The listing builds one solid part. Answer for the finished solid, in the listing's coordinates (mm). Face numbers are marked on the shaded views. A direction names the side the tool comes from. Coordinates: 2 decimals unless noted, no trailing zeros. Order: outer loops, then holes, each group sorted by start corner. A loop starts at its lowest first (then second) coordinate and runs counter-clockwise, first axis right, second up. Notation, with made-up numbers: (84.25, 76) -> (90.25, 76) arc R15 ccw to (90.25, 87) -> close; hole circle Ø4 at (69, -2.5). An arc over 180 degrees is marked (long way). Put each result on its own line as item: value. Start each with the question number.
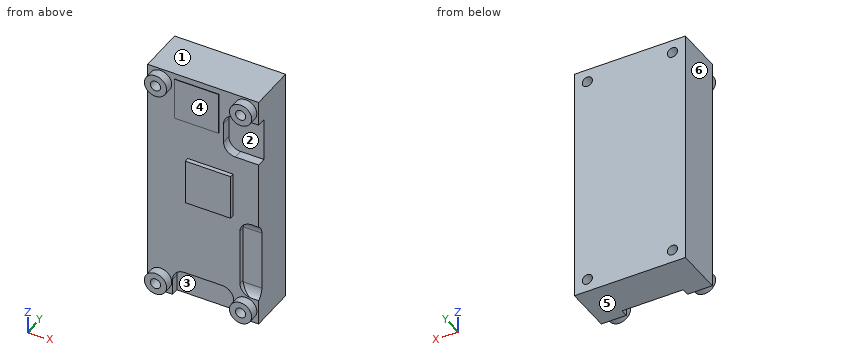
Autodesk Inventor part; units mm, degrees
ref_plane "YZ Plane" through (0, 0, 0) normal (1, 0, 0) x (0, 1, 0)
ref_plane "XZ Plane" through (0, 0, 0) normal (0, 1, 0) x (-1, 0, 0)
ref_plane "XY Plane" through (0, 0, 0) normal (0, 0, 1) x (1, 0, 0)
sketch "Sketch1" plane through (0, 0, 0) normal (0, 1, 0) x (-1, 0, 0)
  line L0 (15, 32.5) -> (-15, 32.5)
  line L1 (-15, 32.5) -> (-15, -32.5)
  line L2 (-15, -32.5) -> (15, -32.5)
  line L3 (15, -32.5) -> (15, 32.5)
  point P0 (0, 0)
  dimension "d0" = 65
  dimension "d1" = 30
  dimension "d2" = 15
  dimension "d3" = 32.5
extrude "Extrusion1" add sketch "Sketch1" along normal blind 12.7
sketch "Sketch2" plane through (0, 0, 0) normal (0, -1, 0) x (1, 0, 0)
  line L0 (8.07, 8.904) -> (-4.13, 8.904)
  line L1 (-4.13, 8.904) -> (-4.13, -3.296)
  line L2 (-4.13, -3.296) -> (8.07, -3.296)
  line L3 (8.07, -3.296) -> (8.07, 8.904)
  line L4 (-15, 32.5) -> (15, 32.5)
  line L5 (15, 32.5) -> (15, -32.5)
  point P0 (0, 0)
  dimension "d6" = 12.2
  dimension "d7" = 12.2
  dimension "d8" = 23.596
  dimension "d9" = 6.93
extrude "Extrusion2" add sketch "Sketch2" along normal blind 1.17
sketch "Sketch3" plane through (0, 0, 0) normal (0, -1, 0) x (1, 0, 0)
  line L0 (15, 32.5) -> (15, -32.5)
  line L1 (15, 25.85) -> (5.5, 25.85)
  line L2 (5.5, 25.85) -> (5.5, 14.15)
  line L3 (5.5, 14.15) -> (15, 14.15)
  line L4 (15, 14.15) -> (15, 25.85)
  line L5 (-15, 32.5) -> (15, 32.5)
  point P0 (0, 0)
  dimension "d12" = 9.5
  dimension "d13" = 11.7
  dimension "d14" = 6.65
extrude "Extrusion3" cut sketch "Sketch3" against normal blind 2.5
sketch "Sketch4" plane through (0, 0, 0) normal (0, -1, 0) x (1, 0, 0)
  line L0 (15, 14.15) -> (15, -32.5)
  line L1 (15, -4.75) -> (10.3, -4.75)
  line L2 (10.3, -4.75) -> (10.3, -13.05)
  line L3 (10.3, -13.05) -> (15, -13.05)
  line L4 (15, -13.05) -> (15, -4.75)
  line L5 (-15, 32.5) -> (15, 32.5)
  point P0 (0, 0)
  dimension "d17" = 4.7
  dimension "d18" = 8.3
  dimension "d19" = 37.25
extrude "Extrusion4" cut sketch "Sketch4" against normal blind 1
sketch "Sketch5" plane through (0, 0, 0) normal (0, -1, 0) x (1, 0, 0)
  line L0 (15, -13.05) -> (15, -32.5)
  line L1 (10.3, -25.65) -> (15, -25.65)
  line L2 (15, -32.5) -> (-15, -32.5)
  line L3 (10.3, -4.75) -> (15, -4.75)
  line L4 (15, -25.65) -> (15, -4.115)
  line L5 (15, -4.115) -> (9.92, -4.115)
  line L6 (9.92, -4.115) -> (9.92, -25.65)
  line L7 (10.3, -25.65) -> (9.92, -25.65)
  point P0 (0, 0)
  point P1 (15, -7.29)
  dimension "d22" = 4.7
  dimension "d24" = 6.85
  dimension "d69" = 5.08
  dimension "d70" = 0.635
extrude "Extrusion5" cut sketch "Sketch5" against normal blind 1.5
sketch "Sketch6" plane through (0, 0, 0) normal (0, -1, 0) x (1, 0, 0)
  circle A0 centre (11.5, 29) radius 3
  circle A1 centre (-11.5, 29) radius 3
  circle A2 centre (-11.5, -29) radius 3
  circle A3 centre (11.5, -29) radius 3
  line L0 (15, -32.5) -> (-15, -32.5)
  line L1 (-15, -32.5) -> (-15, 32.5)
  line L2 (-15, 32.5) -> (15, 32.5)
  point P0 (0, 0)
  dimension "d27" = 6
  dimension "d28" = 6
  dimension "d29" = 6
  dimension "d30" = 6
  dimension "d31" = 0
  dimension "d32" = 23
  dimension "d33" = 58
  dimension "d34" = 3.5
  dimension "d35" = 23
  dimension "d37" = 0
  dimension "d38" = 3.5
  dimension "d42" = 3.5
extrude "Extrusion6" add sketch "Sketch6" along normal blind 2.42
sketch "Sketch7" plane through (11.5, -2.42, 29) normal (0, -1, 0) x (1, 0, 0)
  circle A0 centre (0, 0) radius 3
  circle A1 centre (0, -58) radius 3
  circle A2 centre (-23, -58) radius 3
  circle A3 centre (-23, 0) radius 3
  point P0 (-11.5, -29)
hole "Hole1" at (11.5, -2.42, 29) at (-11.5, -2.42, 29) at (-11.5, -2.42, -29) at (11.5, -2.42, -29) direction (0, 1, 0) diameter 2.75 depth 25.4 tip angle 118
sketch "Sketch8" plane through (0, 0, 0) normal (0, -1, 0) x (1, 0, 0)
  line L0 (15, -32.5) -> (-15, -32.5)
  line L1 (8.255, -32.5) -> (-8.255, -32.5)
  line L2 (-8.255, -32.5) -> (-8.255, -24.88)
  line L3 (-8.255, -24.88) -> (8.255, -24.88)
  line L4 (8.255, -24.88) -> (8.255, -32.5)
  point P0 (0, 0)
  point P1 (0, 0)
  dimension "d50" = 7.62
  dimension "d51" = 16.51
  dimension "d52" = 8.255
extrude "Extrusion7" cut sketch "Sketch8" against normal blind 2.032
sketch "Sketch9" plane through (0, 0, 0) normal (0, -1, 0) x (1, 0, 0)
  line L0 (4.228, 30.9) -> (-7.722, 30.9)
  line L1 (-7.722, 30.9) -> (-7.722, 19.5)
  line L2 (-7.722, 19.5) -> (4.228, 19.5)
  line L3 (4.228, 19.5) -> (4.228, 30.9)
  line L4 (-15, 32.5) -> (15, 32.5)
  line L5 (-15, -32.5) -> (-15, 32.5)
  line L6 (15, 32.5) -> (15, 25.85)
  point P0 (0, 0)
  dimension "d56" = 1.6
  dimension "d57" = 11.4
  dimension "d58" = 11.95
  dimension "d60" = 10.772
extrude "Extrusion9" add sketch "Sketch9" along normal blind 0.1111
fillet "Fillet3" radius 3.175 4 edges at (9.92, 0.75, -25.65) (9.92, 0.75, -4.115) (12.46, 1.5, -4.115) (12.46, 1.5, -25.65)
fillet "Fillet4" radius 3.175 2 edges at (-8.255, 1.016, -24.88) (8.255, 1.016, -24.88)
fillet "Fillet5" radius 3.175 2 edges at (5.5, 1.25, 25.85) (5.5, 1.25, 14.15)
equation "\"d6\" = d7"
equation "\"d28\" = d27"
equation "\"d29\" = d27"
equation "\"d30\" = d27"
equation "\"d35\" = d32"
properties part number "Heat Block for Pi" material "Aluminum 6061"
(1) For a pull along X with two mould halves and no side action, classify the marked faces 4, 5 and 6 as released by +X, released by -X, zero draft, split by the parting line, or undercut.
(2) The part is cut by section D-D on z = -29. Determine the outline of the cut face in (x, y) (3 decimals).
(3) Find the intervals of material crossed by L1, parallel to X at y = 2.25, z = -29 (3 decimals); L2, parallel to Z at x = -11.5, y = 2.25 (3 decimals); L3, parallel to Z at x = 11, y = 3, in increasing order.
(4) A tool of negligible diameter and unlimited length cuts with its end or side. For the marked faces 1, 2 and 3, from which of +Z, -Z, +X, -X, +Y, -Y can it reach the whole face along a straight path? Write none if from no direction.
(5) The part is cut by section A-A on z = 29. Determine the outline of the cut face in (x, y) (3 decimals).
(6) The part is cut by section B-B on x = -11.5. Determine the outline of the cut face in (y, z) (3 decimals).
(7) The part is cut by section C-C on x = 0.5. Determine the outline of the cut face in (y, z), plus the area to 3 significant figures.
(8) Each of these flat-tipped pins is pushed along its axis until it touches: P1, Ø2, axis at x = -11.5, z = 29, coming from the +Y side; P2, Ø0.8, axis at y = 1, z = -13.5, coming from the +X side; P3, Ø9, axis at x = -1.5, z = 26, coming from the -Y side; P4, Ø0.6, axis at x = 3.5, y = -0.5, coming from the -Z side. Where does it stop, or does it pass through?
Worked out:
1. face 4: undercut
1. face 5: zero draft
1. face 6: released by -X
2. outline: (-15, 0) -> (-14.5, 0) -> (-14.5, -2.42) -> (-12.875, -2.42) -> (-12.875, 12.7) -> (-15, 12.7) -> close; (-10.125, -2.42) -> (-8.5, -2.42) -> (-8.5, 0) -> (-8.255, 0) -> (-8.255, 2.032) -> (8.255, 2.032) -> (8.255, 0) -> (8.5, 0) -> (8.5, -2.42) -> (10.125, -2.42) -> (10.125, 12.7) -> (-10.125, 12.7) -> close; (12.875, -2.42) -> (14.5, -2.42) -> (14.5, 0) -> (15, 0) -> (15, 12.7) -> (12.875, 12.7) -> close
3. L1: -15 to -12.875, -10.125 to 10.125, 12.875 to 15
3. L2: -32.5 to -30.375, -27.625 to 27.625, 30.375 to 32.5
3. L3: -32.5 to -30.28, -27.72 to 27.72, 30.28 to 32.5
4. face 1: +Z, +X, -X, +Y, -Y
4. face 2: +X, -Y
4. face 3: -Z, -Y
5. outline: (-15, 0) -> (-14.5, 0) -> (-14.5, -2.42) -> (-12.875, -2.42) -> (-12.875, 12.7) -> (-15, 12.7) -> close; (-10.125, -2.42) -> (-8.5, -2.42) -> (-8.5, 0) -> (-7.722, 0) -> (-7.722, -0.111) -> (4.228, -0.111) -> (4.228, 0) -> (8.5, 0) -> (8.5, -2.42) -> (10.125, -2.42) -> (10.125, 12.7) -> (-10.125, 12.7) -> close; (12.875, -2.42) -> (14.5, -2.42) -> (14.5, 0) -> (15, 0) -> (15, 12.7) -> (12.875, 12.7) -> close
6. outline: (-2.42, -32) -> (0, -32) -> (0, -32.5) -> (12.7, -32.5) -> (12.7, -30.375) -> (-2.42, -30.375) -> close; (-2.42, -27.625) -> (12.7, -27.625) -> (12.7, 27.625) -> (-2.42, 27.625) -> (-2.42, 26) -> (0, 26) -> (0, -26) -> (-2.42, -26) -> close; (-2.42, 30.375) -> (12.7, 30.375) -> (12.7, 32.5) -> (0, 32.5) -> (0, 32) -> (-2.42, 32) -> close
7. outline: (-1.17, -3.3) -> (0, -3.3) -> (0, -24.88) -> (2.03, -24.88) -> (2.03, -32.5) -> (12.7, -32.5) -> (12.7, 32.5) -> (0, 32.5) -> (0, 30.9) -> (-0.11, 30.9) -> (-0.11, 19.5) -> (0, 19.5) -> (0, 8.9) -> (-1.17, 8.9) -> close
7. area: 826 mm2
8. P1: through
8. P2: x = 9.92
8. P3: y = -0.11
8. P4: z = -3.3
